Can you work these out from the model? Positions are in its coordinate system, mm. A direction names the side the tool comes from. Coordinates: 2 decimals unless noted, no trailing zeros. Order: outer loops, then holes, each group sorted by start corner. A loop starts at its lowest first (then second) coordinate and runs counter-clockwise, first axis right, second up. Notation, with made-up numbers: (-38, 62) - (11, 62) arc R13 ccw to (11, 86) - close; hole circle Ø9 at (-1.5, 66.5). An arc over 180 degrees is marked (long way). Return JSON: item names as keys, results as strings. Group by question number.
1) Imagine slicing it at B-B (x = 52). Write out the boundary of the cut face in (y, z), and give its area (3 significant figures).
2) Imagine slicing it at A-A (y = 1.25). Write out the boundary of the cut face in (x, z), and give its area (3 significant figures).
3) Which directions (+Z, -Z, +X, -X, +Y, -Y) give clear straight access to the entire face, cutting with the end or side of a thin tool? Please do faces 1 (the face through (-2, 1, -27)), 2 (the face through (-1, 1, -47)), 3 (the face through (62, 1, 0)).
4) If I drill on line 1 along Z through (x, y) = (63, 0.5); line 2 along X through (y, z) = (1.7, -27.5); line 3 along X through (y, z) = (2.4, -37.5), over which ranges is the centre line in solid material (lowest first)?
5) Imagine slicing it at C-C (z = -29). Write out the boundary of the cut face in (x, y).
6) For pin 1 Ø1.5 at (y, z) = (1, -14) entering from +X; pin 2 Ø1.5 at (x, y) = (-1.5, 2) entering from +Z; pin 3 Ø0.9 at (x, y) = (59, 1) entering from +Z, each with a flat end and sliding along its axis, tell me the tip position at first contact or that it passes through.
```python
from build123d import *

# Parameters (mm, degrees)
SALIENTE_EXTRUIR1_DEPTH = 3


with BuildPart() as part:
    # Croquis1 → Saliente-Extruir1 (new body)
    with BuildSketch(Plane(origin=(0, 0, 0), x_dir=(1, 0, 0), z_dir=(0, 1, 0))):
        Polygon((0, 0), (27, 0), (27, -3), (37, -3), (47, -3), (47, 0), (77, 0), (0, 77), (0, 47), (-3, 47), (-3, 37), (-3, 27), (0, 27), align=None)
    extrude(amount=SALIENTE_EXTRUIR1_DEPTH)


solid = part.part
```
Calculated:
{
 "1": {"outline": "(0, -25) - (3, -25) - (3, 0) - (0, 0) - close", "area": "75.0 mm2"},
 "2": {"outline": "(-3, -47) - (0, -47) - (0, -77) - (77, 0) - (47, 0) - (47, 3) - (27, 3) - (27, 0) - (0, 0) - (0, -27) - (-3, -27) - close", "area": "3,080 mm2"},
 "3": {"face 1": "+Z, -X, +Y, -Y", "face 2": "-Z, -X, +Y, -Y", "face 3": "+Z, +X, +Y, -Y"},
 "4": {"line 1": "-14 to 0", "line 2": "-3 to 49.5", "line 3": "-3 to 39.5"},
 "5": {"outline": "(-3, 0) - (48, 0) - (48, 3) - (-3, 3) - close"},
 "6": {"pin 1": "x = 63.75", "pin 2": "z = -27", "pin 3": "z = 0"}
}
